Read the model definition and answer for the solid it produces. Units are mm, in the model's axes. A direction names the side the tool comes from. Coordinates: 2 decimals unless noted, no trailing zeros. Order: outer loops, then holes, each group sorted by start corner. A loop starts at its lowest first (then second) coordinate and runs counter-clockwise, first axis right, second up.
from build123d import *

# Parameters (mm, degrees)
BOSS_EXTRUDE1_DEPTH = 6.35
SKETCH4_R           = 10.0203
SKETCH4_R_2         = 1.8288
CUT_EXTRUDE3_DEPTH  = 154.060029074


with BuildPart() as part:
    # Sketch2 → Boss-Extrude1 (new body)
    with BuildSketch(Plane.XY):
        with BuildLine():
            Line((-82.55, -6.35), (-82.55, 101.6))
            Line((-82.55, 101.6), (0, 101.6))
            Line((0, 101.6), (0, 95.25))
            ThreePointArc((0, 95.25), (7.439487758, 77.289487758), (25.4, 69.85))
            Line((25.4, 69.85), (114.3, 69.85))
            Line((114.3, 69.85), (114.3, -6.35))
            Line((114.3, -6.35), (-82.55, -6.35))
        make_face()
    extrude(amount=BOSS_EXTRUDE1_DEPTH)

    # Sketch4 → Cut-Extrude3 (cut, through all)
    with BuildSketch(Plane.XY.offset(6.35)):
        with Locations((-42.128660063, 61.122671242)):
            Circle(SKETCH4_R)
        with Locations((-30.224747325, 70.249382672)):
            Circle(SKETCH4_R_2)
        with Locations((-55.984580384, 66.868406363)):
            Circle(SKETCH4_R_2)
        with Locations((-40.176652481, 46.250224691)):
            Circle(SKETCH4_R_2)
    extrude(amount=-CUT_EXTRUDE3_DEPTH, mode=Mode.SUBTRACT)


solid = part.part
Q1. The part is cut by section A-A, the plane z = 1. Determine the outline of the cut face in (x, y).
Q2. The part is cut by section B-B, the plane y = 59. Determine the outline of the cut face in (x, z).
Q3. Determine the mould class of faces 1 (the cylindrical face through (-57.44, 65.76, 3.22)), 2 (the flat face through (17, 36, 6.35)), 3 (the flat face through (-82.55, 47, 3)), 4 (the cylindrical face through (7.24, 77.49, 3.13)) for opening direction X: +X half, -X half, draft (parallel to the pull), parting line (faces both ways), or undercut.
Q4. Straight lines are drawn through the part: L1, parallel to Y at x = 73.5, z = 3.75; L2, parallel to X at y = 94, z = 5; L3, parallel to Y at x = -55, z = 2.75. For each, find the intervals that lie inside material, in ascending order.
Q5. The part is cut by section C-C, the plane x = 55.5. Determine the outline of the cut face in (y, z).
Q6. The part is cut by section D-D, the plane y = 82. Determine the outline of the cut face in (x, z), then the cut area to 3 significant figures.
Q7. Which of the six approach directions +Z, -Z, +X, -X, +Y, -Y give full straight-line access (tool end or side, diameter ignored) to faces 5 (the flat face through (0, 98, 3)), 6 (the flat face through (114.3, 32, 3))?
Q8. Each of these flat-tipped pins is pushed along its axis until it touches: P1, Ø16, axis at x = -42.13, y = 61.12, coming from the -Z side; P2, Ø1, axis at x = 37.5, z = 3.5, coming from the +Y side; P3, Ø1, axis at x = 18.5, z = 1, coming from the +Y side. Where does it stop, or does it pass through?
Computed values:
1. outline: (-82.55, -6.35) - (114.3, -6.35) - (114.3, 69.85) - (25.4, 69.85) arc R25.4 cw to (0, 95.25) - (0, 101.6) - (-82.55, 101.6) - close; hole circle Ø3.66 at (-55.98, 66.87); hole circle Ø20.04 at (-42.13, 61.12); hole circle Ø3.66 at (-40.18, 46.25); hole circle Ø3.66 at (-30.22, 70.25)
2. outline: (-82.55, 0) - (-51.92, 0) - (-51.92, 6.35) - (-82.55, 6.35) - close; (-32.34, 0) - (114.3, 0) - (114.3, 6.35) - (-32.34, 6.35) - close
3. face 1: undercut
3. face 2: draft
3. face 3: -X half
3. face 4: +X half
4. L1: y = -6.35 to 69.85
4. L2: x = -82.55 to 0.03
4. L3: y = -6.35 to 65.33, 68.41 to 101.6
5. outline: (-6.35, 0) - (69.85, 0) - (69.85, 6.35) - (-6.35, 6.35) - close
6. outline: (-82.55, 0) - (3.73, 0) - (3.73, 6.35) - (-82.55, 6.35) - close
6. area: 548 mm2
7. face 5: +Z, -Z, +X, +Y
7. face 6: +Z, -Z, +X, +Y, -Y
8. P1: passes through
8. P2: stops at y = 69.85
8. P3: stops at y = 70.95
